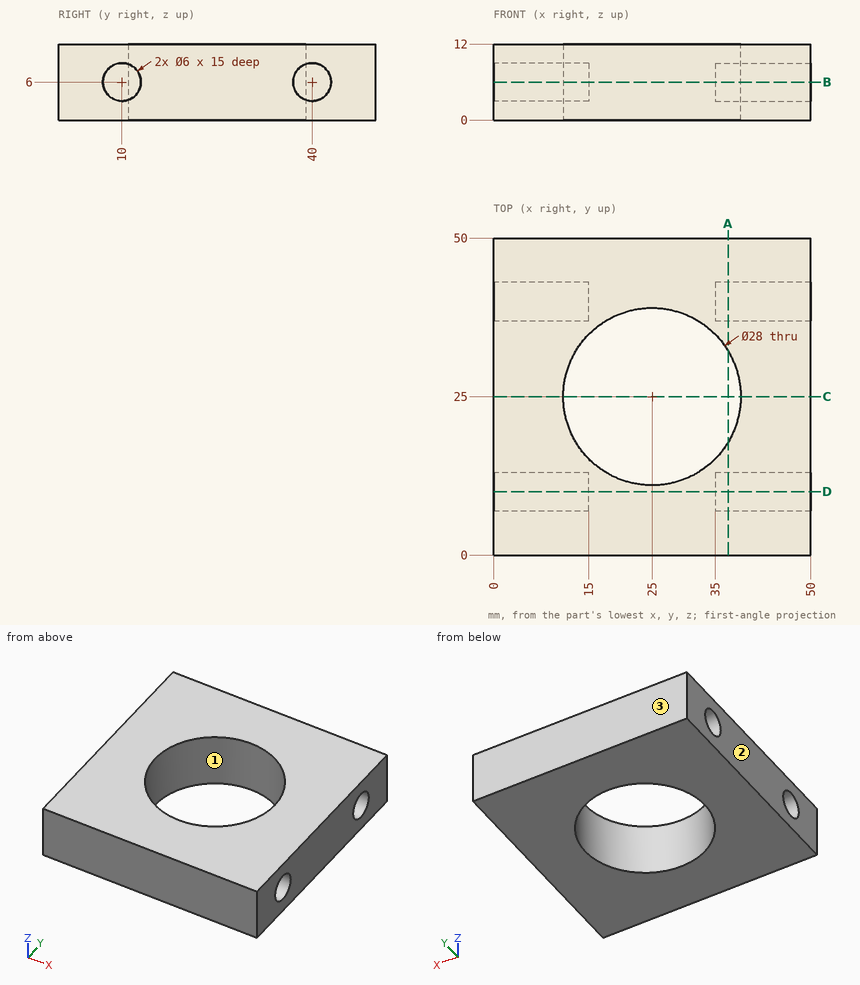
Answer from the drawing. Dimensions are ordinates in mm from the lowest x, y and z of the part. Give positions to 0.01 mm unless a question says otherwise; leave off trailing zeros. Loops run counter-clockwise (first coordinate to the right, second up) from the corner with the lowest first, then second, coordinate; pieces in that order, holes last.
Item 1: Find the intervals of material crossed by line 1 along Y through (x, z) = (10.5, 6.25); line 2 along Y through (x, z) = (44, 8); line 3 along Z through (x, y) = (12.5, 10), in increasing order.
Derived:
line 1: y = 0 to 7.01, 12.99 to 37.01, 42.99 to 50
line 2: y = 0 to 7.76, 12.24 to 37.76, 42.24 to 50
line 3: z = 0 to 3, 9 to 12
Item 2: A cutting plane is placed at B-B (z = 6). Give the vertices of the cut face in (x, y).
Derived:
outline: (0, 0) - (50, 0) - (50, 7) - (35, 7) - (35, 13) - (50, 13) - (50, 37) - (35, 37) - (35, 43) - (50, 43) - (50, 50) - (0, 50) - (0, 43) - (15, 43) - (15, 37) - (0, 37) - (0, 13) - (15, 13) - (15, 7) - (0, 7) - close; hole circle Ø28 at (25, 25)
Item 3: A cutting plane is placed at A-A (x = 37). Give the vertices of the cut face in (y, z), then the cut area to 3 significant figures.
Derived:
outline: (0, 0) - (17.79, 0) - (17.79, 12) - (0, 12) - close; (32.21, 0) - (50, 0) - (50, 12) - (32.21, 12) - close; hole circle Ø6 at (10, 6); hole circle Ø6 at (40, 6)
area: 370 mm2
Item 4: A cutting plane is placed at D-D (y = 10). Give the vertices of the cut face in (x, z).
Derived:
outline: (0, 0) - (50, 0) - (50, 3) - (35, 3) - (35, 9) - (50, 9) - (50, 12) - (0, 12) - (0, 9) - (15, 9) - (15, 3) - (0, 3) - close
Item 5: Determine the mould class of the marked faces 1, 2 and 3 for opening direction X: +X half, -X half, draft (parallel to the pull), parting line (faces both ways), or undercut.
Derived:
face 1: undercut
face 2: -X half
face 3: draft
Item 6: A cutting plane is placed at C-C (y = 25). Give the vertices of the cut face in (x, z), then the cut area to 3 significant figures.
Derived:
outline: (0, 0) - (11, 0) - (11, 12) - (0, 12) - close; (39, 0) - (50, 0) - (50, 12) - (39, 12) - close
area: 264 mm2
Item 7: Each of these flat-tipped pins is pushed along its axis until it touches: pin 1 Ø5.5 at (y, z) = (40, 6) entering from +X; pin 2 Ø22.5 at (x, y) = (25, 25) entering from -Z; pin 3 Ø2 at (x, z) = (12, 4.5) entering from -Y; pin 4 Ø3.5 at (y, z) = (10, 6) entering from -X. Where does it stop, or does it pass through?
Derived:
pin 1: stops at x = 35
pin 2: passes through
pin 3: stops at y = 0
pin 4: stops at x = 15
